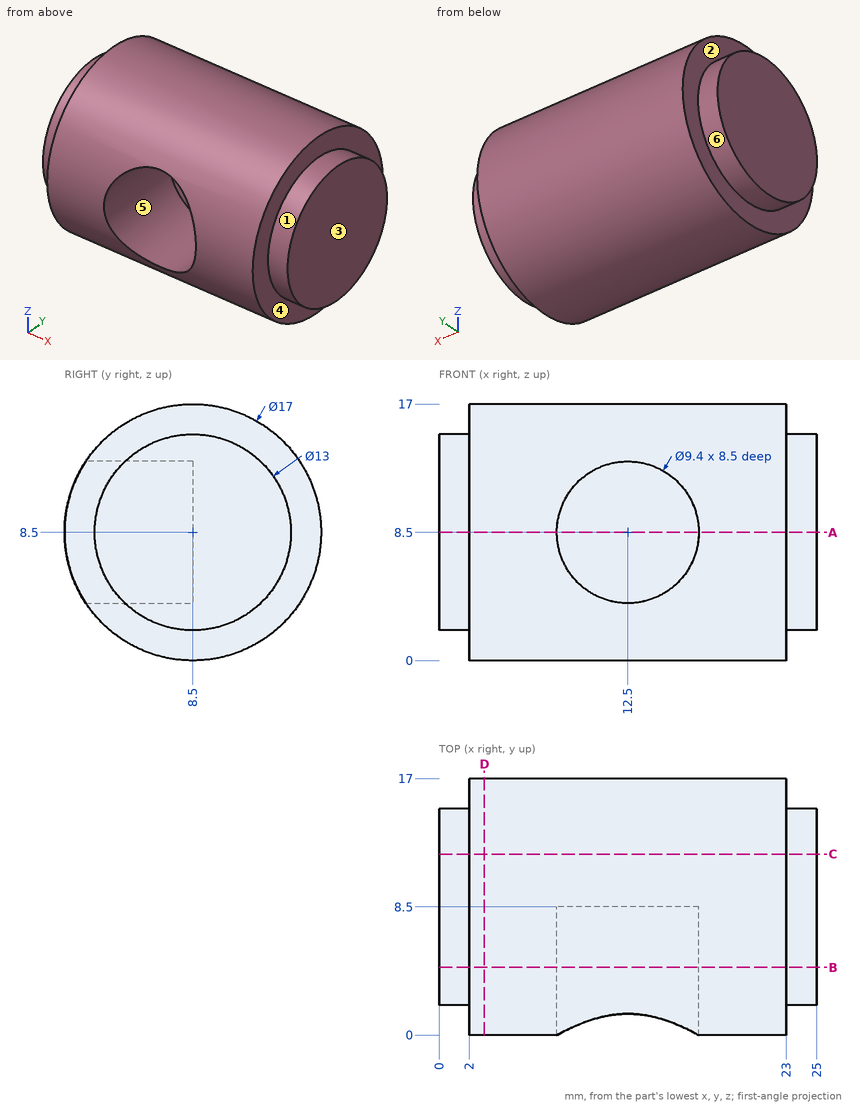
Job drawing, mm, ordinate dimensions from the low corner. One solid piece. A direction names the side the tool comes from. Coordinates: 2 decimals unless noted, no trailing zeros. Write each loop counter-clockwise with the first axis right and the second up, starting at its lowest first coordinate (ties: lowest second). Pieces come first, ordered by that corner, then holes. Notation, with made-up numbers: M 2,-7 L 28,-7 A4 cw 28,0 Z; hole C 3.5,28.25 d5. An arc over 180 degrees is marked long. Answer as a JSON object with one key per item and string values. Group by question number.
1) Pin check, flat tips, straight feed: pin 1 Ø8 at (x, z) = (6.5, 7.5) entering from -Y; pin 2 Ø1.5 at (x, y) = (4, 3.5) entering from -Z; pin 3 Ø3 at (x, y) = (18, 12.5) entering from +Z; pin 4 Ø3 at (x, z) = (12, 9.5) entering from -Y. Stop position of each tip, or through.
2) Saw through at C-C (y = 12). Write the cut outline in (x, z).
3) Saw through at A-A (z = 8.5). Write the cut outline in (x, y).
4) Saw through at B-B (y = 4.5). Write the cut outline in (x, z).
5) Wall check: line 1 (X direction, y = 2.5, z = 8.5); line 2 (X direction, y = 9.5, z = 1.25); line 3 (X direction, y = 3.25, z = 12). Give the ranges that are in metal, low to high. Write a range as from..to.
6) Saw through at D-D (x = 3). Write the cut outline in (y, z).
7) Mould opens along Z. For the marked faces 4, 5 and 6 say: +Z half, -Z half, draft (parallel to the pull), parting line (faces both ways), or undercut.
8) Tool access for the marked faces 1, 2 and 3: list every direction of +Z, -Z, +X, -X, +Y, -Y with a clear straight run to the whole face (end or side of a thin tool).
Values follow:
{
 "1": {"pin 1": "stops at y = 0", "pin 2": "stops at z = 1.14", "pin 3": "stops at z = 16.62", "pin 4": "stops at y = 8.5"},
 "2": {"outline": "M 0,3.02 L 2,3.02 L 2,0.75 L 23,0.75 L 23,3.02 L 25,3.02 L 25,13.98 L 23,13.98 L 23,16.25 L 2,16.25 L 2,13.98 L 0,13.98 Z"},
 "3": {"outline": "M 0,2 L 2,2 L 2,0 L 7.8,0 L 7.8,8.5 L 17.2,8.5 L 17.2,0 L 23,0 L 23,2 L 25,2 L 25,15 L 23,15 L 23,17 L 2,17 L 2,15 L 0,15 Z"},
 "4": {"outline": "M 0,3.38 L 2,3.38 L 2,1 L 23,1 L 23,3.38 L 25,3.38 L 25,13.62 L 23,13.62 L 23,16 L 2,16 L 2,13.62 L 0,13.62 Z; hole C 12.5,8.5 d9.4"},
 "5": {"line 1": "x = 0..7.8, 17.2..25", "line 2": "x = 2..23", "line 3": "x = 0..9.36, 15.64..25"},
 "6": {"outline": "C 8.5,8.5 d17"},
 "7": {"face 4": "draft", "face 5": "undercut", "face 6": "parting line"},
 "8": {"face 1": "+X", "face 2": "-X", "face 3": "+Z, -Z, +X, +Y, -Y"}
}
